Print and shaded views of the part. All mm, measured from the part's lowest x, y and z. A direction names the side the tool comes from. Coordinates: 2 decimals unless noted, no trailing zeros. Loops run counter-clockwise (first coordinate to the right, second up) from the corner with the lowest first, then second, coordinate; pieces in that order, holes last.
1) Saw through at A-A, the plane x = 10. Write the cut outline in (y, z) (3 decimals), and give its area (3 significant figures).
2) Saw through at B-B, the plane z = 10. Write the cut outline in (x, y), and give its area (3 significant figures).
3) Which spindle directions (+Z, -Z, +X, -X, +Y, -Y) get a long thin tool onto all of the face, cutting with end or side? Do the marked faces 1 and 2. Say none if no direction does.
4) Saw through at C-C, the plane y = 2.05. Write the cut outline in (x, z).
5) Pin check, flat tips, straight feed: pin 1 Ø1 at (x, y) = (11.5, 3) entering from -Z; pin 2 Ø4.5 at (x, z) = (16, 10) entering from +Y; pin 3 Ø1.5 at (y, z) = (4, 11) entering from +X; pin 4 Ø5 at (x, z) = (10, 10) entering from +Y. Stop position of each tip, or through.
6) Wall check: line 1 along X through (y, z) = (1.3, 11.25); line 2 along X through (y, z) = (2.5, 4.5) (3 decimals); line 3 along X through (y, z) = (2.5, 3.25) (3 decimals). Give the ranges that are in metal, low to high.
7) Two-plate mould, pull along X, no slides. Class the marked faces 3, 4 and 5: +X half, -X half, draft (parallel to the pull), parting line (faces both ways), or undercut.
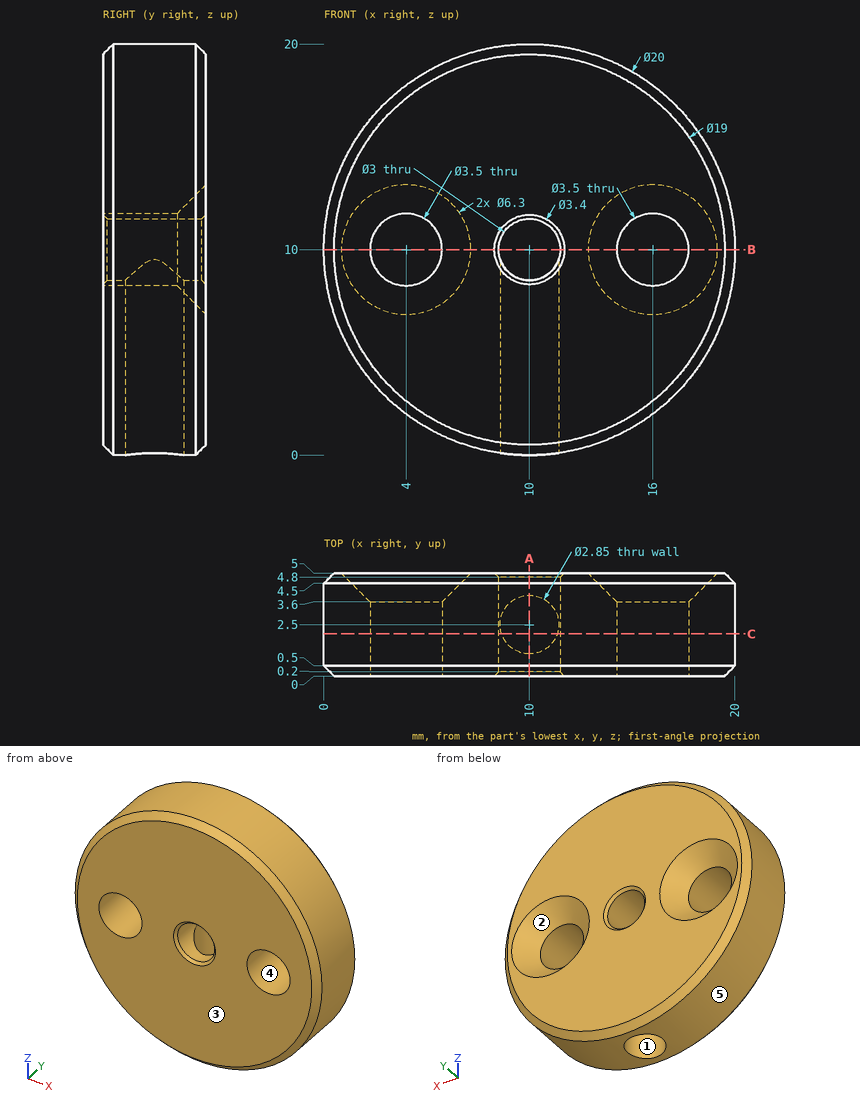
Data:
1. outline: (0, 0.5) - (0.5, 0) - (1.075, 0) - (1.075, 8.5) - (0.2, 8.5) - (0, 8.3) - close; (0, 11.7) - (0.2, 11.5) - (4.8, 11.5) - (5, 11.7) - (5, 19.5) - (4.5, 20) - (0.5, 20) - (0, 19.5) - close; (3.925, 0) - (4.5, 0) - (5, 0.5) - (5, 8.3) - (4.8, 8.5) - (3.925, 8.5) - close
1. area: 60.2 mm2
2. outline: (0, 0.5) - (0.5, 0) - (2.25, 0) - (2.25, 3.6) - (0.85, 5) - (0.5, 5) - (0, 4.5) - close; (5.75, 0) - (8.3, 0) - (8.5, 0.2) - (8.5, 4.8) - (8.3, 5) - (7.15, 5) - (5.75, 3.6) - close; (11.5, 0.2) - (11.7, 0) - (14.25, 0) - (14.25, 3.6) - (12.85, 5) - (11.7, 5) - (11.5, 4.8) - close; (17.75, 0) - (19.5, 0) - (20, 0.5) - (20, 4.5) - (19.5, 5) - (19.15, 5) - (17.75, 3.6) - close
2. area: 45.5 mm2
3. face 1: -Z
3. face 2: +Y
4. outline: (8.65, 0.09) - (8.65, 9.35) arc R1.5 cw (long way) to (11.35, 9.35) - (11.35, 0.09) arc R10 ccw (long way) to start; hole circle Ø3.5 at (4, 10); hole circle Ø3.5 at (16, 10)
5. pin 1: stops at z = 0.07
5. pin 2: stops at y = 4.1
5. pin 3: stops at x = 20
5. pin 4: stops at y = 5
6. line 1: x = 0.08 to 2.78, 5.22 to 9.17, 10.83 to 14.78, 17.22 to 19.92
6. line 2: x = 1.648 to 8.575, 11.425 to 18.352
6. line 3: x = 2.622 to 8.575, 11.425 to 17.378
7. face 3: draft
7. face 4: undercut
7. face 5: parting line
